Part model, mm, in its own coordinate system. A direction names the side the tool comes from. Round coordinates to 2 decimals unless told otherwise and drop trailing zeros. Write each loop counter-clockwise with the first axis right and the second up, starting at its lowest first coordinate (ties: lowest second). Pieces come first, ordered by that corner, then holes. Notation, with made-up numbers: M 81.5,14.25 L 107.5,14.25 A30 ccw 107.5,39.25 Z; hole C 33.5,-35.75 d6. An arc over 180 degrees is marked long. Use a Markdown table: item, result. Add a question column.
1) Drop flat-ended pins along their axis: P1, Ø1.5, axis at y = -36.5, z = 0.5, coming from the +X side; P2, Ø1.5, axis at y = 2, z = 2, coming from the +X side; P3, Ø1.5, axis at x = -78.5, z = 1, coming from the +Y side; P4, Ø12, axis at x = -33.5, y = -56, coming from the -Z side. Give the stop position or say it passes through.
2) Slice it at A-A on x = -1.5. Write the cut outline in (y, z).
3) Slice it at C-C on x = -63. Write the cut outline in (y, z), plus the area to 3 significant figures.
4) Which spindle directions (+Z, -Z, +X, -X, +Y, -Y) get a long thin tool onto all of the face, cutting with end or side? Do faces 3 (the face through (-38, -39, 1)), 4 (the face through (77, -58, 1)), 5 (the face through (-1, -41, 0)). Say none if no direction does.
5) Slice it at B-B on y = -22.5. Write the cut outline in (x, z), plus the area to 3 significant figures.
6) Wall check: probe 1 along X at (y, z) = (-55, 2.75); probe 2 along X at (y, z) = (-49, 1.95); probe 3 along Y at (x, z) = (45.5, 0.35). Give the ranges that are in metal, low to high.
7) Two-plate mould, pull along X, no slides. Class faces 1 (the face through (-52, -58, 1)), 2 (the face through (-1, -41, 3)): released by +X, released by -X, zero draft, split by the parting line, or undercut.
8) Slice it at D-D on z = 1.6. Give the number of separate pieces and of enclosed holes in the cut face, plus the area to 3 significant figures.
Autodesk Inventor part; units mm, degrees
ref_plane "YZ Plane" through (0, 0, 0) normal (1, 0, 0) x (0, 1, 0)
ref_plane "XZ Plane" through (0, 0, 0) normal (0, 1, 0) x (-1, 0, 0)
ref_plane "XY Plane" through (0, 0, 0) normal (0, 0, 1) x (1, 0, 0)
sketch "Sketch1" plane through (0, 0, 0) normal (0, 0, 1) x (1, 0, 0)
  line L0 (-40, 0) -> (-40, -35)
  line L1 (-35, -40) -> (35, -40)
  line L2 (40, -35) -> (40, 0)
  line L3 (104, -70) -> (-104, -70)
  line L4 (-60, 0) -> (-60, 3)
  line L5 (-60, 3) -> (-70, 3)
  line L6 (-70, 3) -> (-70, 0)
  line L7 (-90, 0) -> (-70, 0)
  line L8 (-60, 0) -> (-40, 0)
  line L9 (70, 0) -> (70, 3)
  line L10 (70, 3) -> (60, 3)
  line L11 (60, 3) -> (60, 0)
  line L12 (40, 0) -> (60, 0)
  line L13 (70, 0) -> (90, 0)
  arc A0 (-105, -69) -> (-104, -70) centre (-104, -69) ccw
  arc A1 (104, -70) -> (105, -69) centre (104, -69) ccw
  line L14 (-90, -40) -> (-84, -40)
  line L15 (-84, -40) -> (-84, -50)
  line L16 (90, -40) -> (84, -40)
  line L17 (84, -40) -> (84, -50)
  line L18 (-43.5, -10) -> (-46.5, -10)
  line L19 (-46.5, -10) -> (-46.5, -20)
  line L20 (-46.5, -20) -> (-43.5, -20)
  line L21 (-43.5, -20) -> (-43.5, -10)
  line L22 (43.5, -10) -> (46.5, -10)
  line L23 (46.5, -10) -> (46.5, -20)
  line L24 (46.5, -20) -> (43.5, -20)
  line L25 (43.5, -20) -> (43.5, -10)
  line L26 (-46.5, -50) -> (-43.5, -50)
  line L27 (-43.5, -50) -> (-43.5, -60)
  line L28 (-43.5, -60) -> (-46.5, -60)
  line L29 (-46.5, -60) -> (-46.5, -50)
  line L30 (43.5, -50) -> (46.5, -50)
  line L31 (46.5, -50) -> (46.5, -60)
  line L32 (46.5, -60) -> (43.5, -60)
  line L33 (43.5, -60) -> (43.5, -50)
  line L34 (-5, -53) -> (5, -53)
  line L35 (5, -53) -> (5, -56)
  line L36 (5, -56) -> (-5, -56)
  line L37 (-5, -56) -> (-5, -53)
  line L38 (-100, -40) -> (-100, -20)
  line L39 (-100, -20) -> (-92, -20)
  line L40 (-90, -40) -> (-90, -50)
  line L41 (90, -40) -> (90, -50)
  line L42 (90, -50) -> (84, -50)
  line L43 (100, -40) -> (100, -20)
  line L44 (100, -20) -> (92, -20)
  line L45 (90, -18) -> (90, 0)
  line L46 (-90, 0) -> (-90, -18)
  arc A2 (-92, -20) -> (-90, -18) centre (-92, -18) ccw
  arc A3 (90, -18) -> (92, -20) centre (92, -18) ccw
  line L47 (-90, -50) -> (-84, -50)
  line L48 (-100, -40) -> (-104, -40)
  line L49 (100, -40) -> (104, -40)
  arc A4 (-104, -40) -> (-105, -41) centre (-104, -41) ccw
  arc A5 (105, -41) -> (104, -40) centre (104, -41) ccw
  line L50 (-104, -50) -> (-100, -50)
  line L51 (-100, -50) -> (-100, -60)
  line L52 (-100, -60) -> (-104, -60)
  line L53 (-105, -69) -> (-105, -61)
  line L54 (-105, -49) -> (-105, -41)
  arc A6 (-104, -60) -> (-105, -61) centre (-104, -61) ccw
  arc A7 (-105, -49) -> (-104, -50) centre (-104, -49) ccw
  line L55 (104, -50) -> (100, -50)
  line L56 (100, -50) -> (100, -60)
  line L57 (100, -60) -> (104, -60)
  line L58 (105, -41) -> (105, -49)
  line L59 (105, -61) -> (105, -69)
  arc A8 (105, -61) -> (104, -60) centre (104, -61) ccw
  arc A9 (104, -50) -> (105, -49) centre (104, -49) ccw
  arc A10 (-40, -35) -> (-35, -40) centre (-35, -35) ccw
  arc A11 (35, -40) -> (40, -35) centre (35, -35) ccw
  line L60 (-73, -10) -> (-56, -10)
  line L61 (-51, -15) -> (-51, -55)
  line L62 (-56, -60) -> (-73, -60)
  line L63 (-78, -55) -> (-78, -15)
  line L64 (56, -10) -> (73, -10)
  line L65 (78, -15) -> (78, -55)
  line L66 (73, -60) -> (56, -60)
  line L67 (51, -55) -> (51, -15)
  arc A12 (-73, -10) -> (-78, -15) centre (-73, -15) ccw
  arc A13 (-51, -15) -> (-56, -10) centre (-56, -15) ccw
  arc A14 (-56, -60) -> (-51, -55) centre (-56, -55) ccw
  arc A15 (-78, -55) -> (-73, -60) centre (-73, -55) ccw
  arc A16 (56, -10) -> (51, -15) centre (56, -15) ccw
  arc A17 (78, -15) -> (73, -10) centre (73, -15) ccw
  arc A18 (73, -60) -> (78, -55) centre (73, -55) ccw
  arc A19 (51, -55) -> (56, -60) centre (56, -55) ccw
  point P0 (0, 0)
  point P1 (105, -70)
  point P2 (-105, -70)
  point P3 (-90, -20)
  point P4 (90, -20)
  point P5 (-105, -40)
  point P6 (105, -50)
  point P7 (-40, -40)
  point P8 (40, -40)
  dimension "d0" = 80
  dimension "d1" = 40
  dimension "d2" = 50
  dimension "d10" = 50
  dimension "d15" = 3
  dimension "d16" = 10
  dimension "d18" = 10
  dimension "d20" = 3
  dimension "d23" = 40
  dimension "d24" = 40
  dimension "d27" = 1
  dimension "d28" = 10
  dimension "d29" = 6
  dimension "d31" = 40
  dimension "d32" = 10
  dimension "d33" = 6
  dimension "d35" = 40
  dimension "d39" = 10
  dimension "d40" = 3
  dimension "d41" = 10
  dimension "d42" = 3
  dimension "d44" = 10
  dimension "d45" = 10
  dimension "d50" = 3
  dimension "d51" = 10
  dimension "d52" = 10
  dimension "d54" = 3
  dimension "d55" = 10
  dimension "d56" = 10
  dimension "d60" = 10
  dimension "d61" = 3
  dimension "d62" = 17
  dimension "d66" = 40
  dimension "d67" = 40
  dimension "d71" = 3.5
  dimension "d72" = 3.5
  dimension "d73" = 3.5
  dimension "d74" = 3.5
  dimension "d77" = 20
  dimension "d78" = 20
  dimension "d79" = 10
  dimension "d80" = 10
  dimension "d81" = 2
  dimension "d82" = 10
  dimension "d84" = 50
  dimension "d85" = 20
  dimension "d86" = 20
  dimension "d87" = 60
  dimension "d88" = 5
  dimension "d92" = 30
  dimension "d93" = 5
  dimension "d94" = 30
  dimension "d95" = 1
  dimension "d97" = 10
  dimension "d98" = 10
  dimension "d99" = 1
  dimension "d100" = 10
  dimension "d101" = 10
  dimension "d102" = 5
  dimension "d103" = 5
  dimension "d104" = 210
  dimension "d105" = 1
  dimension "d106" = 5
  dimension "d107" = 70
extrude "Extrusion8" add sketch "Sketch1" along normal blind 3
properties part number "Bulkhead 25083113"
Entries:
| question | item | result |
|---|---|---|
| 1 | P1 | stops at x = 100 |
| 1 | P2 | stops at x = 70 |
| 1 | P3 | stops at y = 0 |
| 1 | P4 | stops at z = 0 |
| 2 | outline | M -70,0 L -56,0 L -56,3 L -70,3 Z; M -53,0 L -40,0 L -40,3 L -53,3 Z |
| 3 | outline | M -70,0 L -60,0 L -60,3 L -70,3 Z; M -10,0 L 3,0 L 3,3 L -10,3 Z |
| 3 | area | 69.0 mm^2 |
| 4 | face 3 | +Z, -Z, +Y |
| 4 | face 4 | +Z, -Z |
| 4 | face 5 | -Z, +X, -X, +Y, -Y |
| 5 | outline | M -100,0 L -78,0 L -78,3 L -100,3 Z; M -51,0 L -40,0 L -40,3 L -51,3 Z; M 40,0 L 51,0 L 51,3 L 40,3 Z; M 78,0 L 100,0 L 100,3 L 78,3 Z |
| 5 | area | 198 mm^2 |
| 6 | probe 1 | x = -100 to -78, -51 to -46.5, -43.5 to -5, 5 to 43.5, 46.5 to 51, 78 to 100 |
| 6 | probe 2 | x = -105 to -90, -84 to -78, -51 to 51, 78 to 84, 90 to 105 |
| 6 | probe 3 | y = -70 to -60, -50 to -20, -10 to 0 |
| 7 | face 1 | undercut |
| 7 | face 2 | zero draft |
| 8 | separate pieces | 1 |
| 8 | enclosed holes | 9 |
| 8 | area | 7,740 mm^2 |
